```python
from build123d import *

# Parameters (mm, degrees)
MODEL_R                  = 1.8
RESSALTO_EXTRUS_O1_DEPTH = 6


with BuildPart() as part:
    # Model → Ressalto-extrusão1 (new body)
    with BuildSketch(Plane.XY):
        Polygon((53.041414253, 36.88413465), (53.455627815, 37.201971895), (53.937989725, 37.40177274), (54.455627815, 37.469921087), (59.255622257, 37.469921087), (59.773260347, 37.40177274), (60.255622257, 37.201971895), (60.66983582, 36.88413465), (60.987673065, 36.469921087), (61.18747391, 35.987559177), (61.255622257, 35.469921087), (61.255622257, 31.119923196), (64.255622257, 31.119923196), (64.255622257, 10.119923196), (60.255622257, 6.119923196), (29.655637917, 6.119923196), (25.655637917, 10.119923196), (25.655637917, 31.119923196), (28.655637917, 31.119923196), (28.655637917, 35.469921087), (28.723786264, 35.987559177), (28.923587109, 36.469921087), (29.241424354, 36.88413465), (29.655637917, 37.201971895), (30.137999826, 37.40177274), (30.655637917, 37.469921087), (35.455633882, 37.469921087), (35.973271972, 37.40177274), (36.455633882, 37.201971895), (36.869847444, 36.88413465), (37.187684689, 36.469921087), (37.387485534, 35.987559177), (37.455633882, 35.469921087), (37.455633882, 31.119923196), (42.755625888, 31.119923196), (42.755625888, 25.819924374), (40.955627657, 25.819924374), (40.955627657, 20.71992661), (42.755625888, 20.71992661), (42.755625888, 16.769926787), (47.15563056, 16.769926787), (47.15563056, 20.71992661), (48.955628792, 20.71992661), (48.955628792, 25.819924374), (47.15563056, 25.819924374), (47.15563056, 31.119923196), (52.455627815, 31.119923196), (52.455627815, 35.469921087), (52.523776162, 35.987559177), (52.723577008, 36.469921087), align=None)
        with Locations((56.255622257, 17.119923196)):
            Circle(MODEL_R, mode=Mode.SUBTRACT)
        with Locations((33.655637917, 17.119923196)):
            Circle(MODEL_R, mode=Mode.SUBTRACT)
    extrude(amount=RESSALTO_EXTRUS_O1_DEPTH)


solid = part.part
```
Geometry check sheet. Reference: the model listing, model coordinates, mm. A direction names the side the tool comes from. Give positions to 0.01 mm unless a question says otherwise; leave off trailing zeros. Loops run counter-clockwise (first coordinate to the right, second up) from the corner with the lowest first, then second, coordinate; pieces in that order, holes last. Notation, with made-up numbers: M -25,16.25 L 32,16.25 A20 ccw 32,45.25 Z; hole C 74.5,-33.5 d3. An arc over 180 degrees is marked long. Write item = value, one per line. Start each with the question number.
1. Tool access check on faces 5 (the face through (41, 19, 0)), 6 (the face through (52.456, 33, 3)), 7 (the face through (48, 20.72, 3)), 8 (the face through (63, 31.12, 3)), 9 (the face through (33, 37.47, 3)). Record the directions out of +Z, -Z, +X, -X, +Y, -Y that give a thin tool (end or side, any length) a straight path to the whole face; none if there is none.
2. Section check A-A, the plane x = 42. Enter the section's corners in (y, z), plus the area to 3 significant figures.
3. Section check D-D, the plane x = 28. Enter the section's corners in (y, z), plus the area to 3 significant figures.
4. Thickness scan on probe 1 along X at (y, z) = (25, 1.95); probe 2 along X at (y, z) = (36, 1.25); probe 3 along X at (y, z) = (18, 3.7). Record the ranges inside material, lowest first.
5. Section check C-C, the plane z = 5. Give the number of separate pieces and of enclosed holes in the cut face, plus the area to 3 significant figures.
6. Draft check along X on faces 1 (the face through (50, 31.12, 3)), 2 (the face through (42.756, 19, 3)), 3 (the face through (61.256, 33, 3)), 4 (the face through (27.684, 8.092, 2.958)). Enter one of: +X half, -X half, draft (parallel to the pull), parting line (faces both ways), or undercut.
7. Go/stop test with flat-tipped pins: P1, Ø3.5, axis at y = 33, z = 3, coming from the +X side; P2, Ø3, axis at x = 48.5, z = 1.5, coming from the +Y side; P3, Ø1, axis at x = 53, z = 1, coming from the +Y side. Record where each tip stops, or that it passes through.
8. Section check B-B, the plane y = 34. Enter the section's corners in (x, z).
Values follow:
q1.face_5 = -Z, +X, -X, +Y, -Y
q1.face_6 = +Z, -Z, +Y
q1.face_7 = +Z, -Z
q1.face_8 = +Z, -Z, +X, +Y
q1.face_9 = +Z, -Z, +X, -X, +Y
q2.outline = M 6.12,0 L 20.72,0 L 20.72,6 L 6.12,6 Z; M 25.82,0 L 31.12,0 L 31.12,6 L 25.82,6 Z
q2.area = 119 mm^2
q3.outline = M 7.78,0 L 31.12,0 L 31.12,6 L 7.78,6 Z
q3.area = 140 mm^2
q4.probe_1 = 25.66 to 40.96, 48.96 to 64.26
q4.probe_2 = 28.73 to 37.38, 52.53 to 61.18
q4.probe_3 = 25.66 to 32.09, 35.23 to 42.76, 47.16 to 54.69, 57.83 to 64.26
q5.separate_pieces = 1
q5.enclosed_holes = 2
q5.area = 955 mm^2
q6.face_1 = undercut
q6.face_2 = undercut
q6.face_3 = +X half
q6.face_4 = -X half
q7.P1 = 61.26
q7.P2 = 31.12
q7.P3 = 37.22
q8.outline = M 28.66,0 L 37.46,0 L 37.46,6 L 28.66,6 Z; M 52.46,0 L 61.26,0 L 61.26,6 L 52.46,6 Z
